Work out the finished part from the listing and answer in its coordinate system (mm). A direction names the side the tool comes from. Coordinates: 2 decimals unless noted, no trailing zeros. Order: outer loops, then holes, each group sorted by start corner. A loop starts at its lowest first (then second) coordinate and runs counter-clockwise, first axis right, second up.
1. A tool of negligible diameter and unlimited length cuts with its end or side. For faces 3 (the flat face through (1.7, 0.5, 5.08)), 4 (the flat face through (0, 0.5, 2.5)), from which of +Z, -Z, +X, -X, +Y, -Y can it reach the whole face along a straight path? Write none if from no direction.
2. Find the intervals of material crossed by probe 1 along Z at (x, y) = (1, 1.5) (3 decimals); probe 2 along Y at (x, z) = (0.4, 2.9); probe 3 along X at (y, z) = (0.15, 3.95), in increasing order.
3. Flat-ended cylindrical pins translate along their axes: pin 1 Ø0.6 at (x, y) = (0.5, -0.5) entering from +Z (3 decimals); pin 2 Ø1.1 at (y, z) = (0.5, 3.5) entering from +X. Find the tip coordinate at first contact, or state that the pin passes through.
4. The part is cut by section A-A, the plane y = 3.4. Count the separate pieces of the cut face and the enclosed holes in it, then the cut area to 3 significant figures.
5. Determine the mould class of faces 1 (the flat face through (1.7, 0, 2.5)), 2 (the flat face through (3.4, 0.5, 2.5)) for opening direction Y: +Y half, -Y half, draft (parallel to the pull), parting line (faces both ways), or undercut.
6. The part is cut by section C-C, the plane z = 4.75. Give the vertices of the cut face in (x, y).
7. The part is cut by section D-D, the plane x = 1.8. Give the vertices of the cut face in (y, z), then the cut area to 3 significant figures.
8. The part is cut by section B-B, the plane x = 4.05. Give the vertices of the cut face in (y, z) (3 decimals).
```python
from build123d import *

# Parameters (mm, degrees)
SKIZZE1_W                         = 3.4
SKIZZE1_H                         = 1
AUFSATZ_LINEAR_AUSTRAGEN1_DEPTH   = 1.27
SKIZZE3_W                         = 0.4
SKIZZE3_H                         = 0.4
AUFSATZ_LINEAR_AUSTRAGEN3_DEPTH   = 0.5
SKIZZE4_W                         = 0.4
SKIZZE4_H                         = 0.4
AUFSATZ_LINEAR_AUSTRAGEN4_DEPTH   = 1.915
SKIZZE5_W                         = 0.4
SKIZZE5_H                         = 0.4
AUFSATZ_LINEAR_AUSTRAGEN5_DEPTH   = 1.915
SKIZZE6_W                         = 0.4
SKIZZE6_H                         = 0.4
AUFSATZ_LINEAR_AUSTRAGEN6_DEPTH   = 3
FASE2_SIZE                        = 0.1
VERRUNDUNG1_R                     = 0.1
VERRUNDUNG2_R                     = 0.4
LINEARES_MUSTER1_COUNT            = 4
LINEARES_MUSTER1_PITCH            = 1.27
FASE2_OF_LINEARES_MUSTER1_SIZE    = 0.1
VERRUNDUNG1_OF_LINEARES_MUSTER1_R = 0.1
VERRUNDUNG2_OF_LINEARES_MUSTER1_R = 0.4


with BuildPart() as part:
    # Skizze1 → Aufsatz-Linear austragen1 (new body)
    with BuildSketch(Plane.XY):
        with Locations((1.7, 0.5)):
            Rectangle(SKIZZE1_W, SKIZZE1_H)
    aufsatz_linear_austragen1 = extrude(amount=AUFSATZ_LINEAR_AUSTRAGEN1_DEPTH)

    # Skizze3 → Aufsatz-Linear austragen3 (add)
    with BuildSketch(Plane.XZ):
        with Locations((1.065, 0.635)):
            Rectangle(SKIZZE3_W, SKIZZE3_H)
        with Locations((2.335, 0.635)):
            Rectangle(SKIZZE3_W, SKIZZE3_H)
    aufsatz_linear_austragen3 = extrude(amount=AUFSATZ_LINEAR_AUSTRAGEN3_DEPTH)

    # Skizze4 → Aufsatz-Linear austragen4 (add)
    with BuildSketch(Plane(origin=(2.535, 0, 0), x_dir=(0, 0, -1), z_dir=(1, 0, 0))):
        with Locations((-0.635, -0.3)):
            Rectangle(SKIZZE4_W, SKIZZE4_H)
    aufsatz_linear_austragen4 = extrude(amount=AUFSATZ_LINEAR_AUSTRAGEN4_DEPTH)

    # Skizze5 → Aufsatz-Linear austragen5 (add)
    with BuildSketch(Plane.ZY.offset(-0.865)):
        with Locations((0.635, -0.3)):
            Rectangle(SKIZZE5_W, SKIZZE5_H)
    aufsatz_linear_austragen5 = extrude(amount=AUFSATZ_LINEAR_AUSTRAGEN5_DEPTH)

    # Skizze6 → Aufsatz-Linear austragen6 (add)
    with BuildSketch(Plane(origin=(0, 1, 0), x_dir=(1, 0, 0), z_dir=(0, 1, 0))):
        with Locations((1.065, -0.635)):
            Rectangle(SKIZZE6_W, SKIZZE6_H)
        with Locations((2.335, -0.635)):
            Rectangle(SKIZZE6_W, SKIZZE6_H)
    aufsatz_linear_austragen6 = extrude(amount=AUFSATZ_LINEAR_AUSTRAGEN6_DEPTH)

    # Fase2
    fase2_edges = [part.edges().sort_by_distance(p)[0] for p in [
        (4.45, -0.3, 0.835),
        (4.45, -0.5, 0.635),
        (4.45, -0.3, 0.435),
        (4.45, -0.1, 0.635),
        (-1.05, -0.3, 0.835),
        (-1.05, -0.1, 0.635),
        (-1.05, -0.3, 0.435),
        (-1.05, -0.5, 0.635),
        (1.265, 4, 0.635),
        (1.065, 4, 0.435),
        (0.865, 4, 0.635),
        (1.065, 4, 0.835),
        (2.535, 4, 0.635),
        (2.335, 4, 0.435),
        (2.135, 4, 0.635),
        (2.335, 4, 0.835),
    ]]
    chamfer(fase2_edges, length=FASE2_SIZE)

    # Verrundung1
    verrundung1_edges = [part.edges().sort_by_distance(p)[0] for p in [
        (0.865, -0.1, 0.635),
        (2.535, -0.1, 0.635),
    ]]
    fillet(verrundung1_edges, radius=VERRUNDUNG1_R - 0.0001)  # a hair under: the kernel refuses the full size

    # Verrundung2
    verrundung2_edges = [part.edges().sort_by_distance(p)[0] for p in [
        (1.265, -0.5, 0.635),
        (2.135, -0.5, 0.635),
    ]]
    fillet(verrundung2_edges, radius=VERRUNDUNG2_R)

    # Lineares Muster1: Aufsatz-Linear austragen1, Aufsatz-Linear austragen3, Aufsatz-Linear austragen4, Aufsatz-Linear austragen5, Aufsatz-Linear austragen6 ×4
    with Locations(*[(0, 0, i * LINEARES_MUSTER1_PITCH) for i in range(1, LINEARES_MUSTER1_COUNT)]):
        add(aufsatz_linear_austragen1)
        add(aufsatz_linear_austragen3)
        add(aufsatz_linear_austragen4)
        add(aufsatz_linear_austragen5)
        add(aufsatz_linear_austragen6)

    # Fase2 of Lineares Muster1
    fase2_of_lineares_muster1_edges = [part.edges().sort_by_distance(p)[0] for p in [
        (4.45, -0.3, 2.105),
        (4.45, -0.5, 1.905),
        (4.45, -0.3, 1.705),
        (4.45, -0.1, 1.905),
        (-1.05, -0.3, 2.105),
        (-1.05, -0.1, 1.905),
        (-1.05, -0.3, 1.705),
        (-1.05, -0.5, 1.905),
        (1.265, 4, 1.905),
        (1.065, 4, 1.705),
        (0.865, 4, 1.905),
        (1.065, 4, 2.105),
        (2.535, 4, 1.905),
        (2.335, 4, 1.705),
        (2.135, 4, 1.905),
        (2.335, 4, 2.105),
        (4.45, -0.3, 3.375),
        (4.45, -0.5, 3.175),
        (4.45, -0.3, 2.975),
        (4.45, -0.1, 3.175),
        (-1.05, -0.3, 3.375),
        (-1.05, -0.1, 3.175),
        (-1.05, -0.3, 2.975),
        (-1.05, -0.5, 3.175),
        (1.265, 4, 3.175),
        (1.065, 4, 2.975),
        (0.865, 4, 3.175),
        (1.065, 4, 3.375),
        (2.535, 4, 3.175),
        (2.335, 4, 2.975),
        (2.135, 4, 3.175),
        (2.335, 4, 3.375),
        (4.45, -0.3, 4.645),
        (4.45, -0.5, 4.445),
        (4.45, -0.3, 4.245),
        (4.45, -0.1, 4.445),
        (-1.05, -0.3, 4.645),
        (-1.05, -0.1, 4.445),
        (-1.05, -0.3, 4.245),
        (-1.05, -0.5, 4.445),
        (1.265, 4, 4.445),
        (1.065, 4, 4.245),
        (0.865, 4, 4.445),
        (1.065, 4, 4.645),
        (2.535, 4, 4.445),
        (2.335, 4, 4.245),
        (2.135, 4, 4.445),
        (2.335, 4, 4.645),
    ]]
    chamfer(fase2_of_lineares_muster1_edges, length=FASE2_OF_LINEARES_MUSTER1_SIZE)

    # Verrundung1 of Lineares Muster1
    verrundung1_of_lineares_muster1_edges = [part.edges().sort_by_distance(p)[0] for p in [
        (0.865, -0.1, 1.905),
        (2.535, -0.1, 1.905),
        (0.865, -0.1, 3.175),
        (2.535, -0.1, 3.175),
        (0.865, -0.1, 4.445),
        (2.535, -0.1, 4.445),
    ]]
    fillet(verrundung1_of_lineares_muster1_edges, radius=VERRUNDUNG1_OF_LINEARES_MUSTER1_R - 0.0001)  # a hair under: the kernel refuses the full size

    # Verrundung2 of Lineares Muster1
    verrundung2_of_lineares_muster1_edges = [part.edges().sort_by_distance(p)[0] for p in [
        (1.265, -0.5, 1.905),
        (2.135, -0.5, 1.905),
        (1.265, -0.5, 3.175),
        (2.135, -0.5, 3.175),
        (1.265, -0.5, 4.445),
        (2.135, -0.5, 4.445),
    ]]
    fillet(verrundung2_of_lineares_muster1_edges, radius=VERRUNDUNG2_OF_LINEARES_MUSTER1_R)


solid = part.part
```
Geometry says:
1. face 3: +Z, +X, -X, +Y, -Y
1. face 4: +Z, -Z, -X, +Y
2. probe 1: z = 0.435 to 0.835, 1.705 to 2.105, 2.975 to 3.375, 4.245 to 4.645
2. probe 2: y = 0 to 1
2. probe 3: x = 0 to 3.4
3. pin 1: stops at z = 4.645
3. pin 2: stops at x = 3.4
4. separate pieces: 8
4. enclosed holes: 0
4. area: 1.28 mm2
5. face 1: undercut
5. face 2: draft
6. outline: (0, 0) - (3.4, 0) - (3.4, 1) - (0, 1) - close
7. outline: (0, 0) - (1, 0) - (1, 5.08) - (0, 5.08) - close
7. area: 5.08 mm2
8. outline: (-0.5, 0.435) - (-0.1, 0.435) - (-0.1, 0.835) - (-0.5, 0.835) - close; (-0.5, 1.705) - (-0.1, 1.705) - (-0.1, 2.105) - (-0.5, 2.105) - close; (-0.5, 2.975) - (-0.1, 2.975) - (-0.1, 3.375) - (-0.5, 3.375) - close; (-0.5, 4.245) - (-0.1, 4.245) - (-0.1, 4.645) - (-0.5, 4.645) - close
